from build123d import *

# Parameters (mm, degrees)
SKETCH1_R           = 25
BOSS_EXTRUDE1_DEPTH = 10
SKETCH2_R           = 1.6
CUT_EXTRUDE1_DEPTH  = 37.742346142
SKETCH5_R           = 2.85
CUT_EXTRUDE4_DEPTH  = 3.2
CIRPATTERN1_COUNT   = 4
SKETCH8_R           = 1.6
CUT_EXTRUDE6_DEPTH  = 37.742346142
CUT_EXTRUDE2_DEPTH  = 2.6
CIRPATTERN2_COUNT   = 4
SKETCH4_R           = 7
CUT_EXTRUDE3_DEPTH  = 37.742346142
SKETCH6_R           = 1.6
CUT_EXTRUDE5_DEPTH  = 37.742346142
CIRPATTERN3_COUNT   = 4


with BuildPart() as part:
    # Sketch1 → Boss-Extrude1 (new body)
    with BuildSketch(Plane.XY):
        Circle(SKETCH1_R)
    extrude(amount=BOSS_EXTRUDE1_DEPTH)

    # Sketch2 → Cut-Extrude1 (cut, through all)
    with BuildSketch(Plane.XY.offset(10)):
        with Locations((-8.838834765, 8.838834765)):
            Circle(SKETCH2_R)
    cut_extrude1 = extrude(amount=-CUT_EXTRUDE1_DEPTH, mode=Mode.SUBTRACT)

    # Sketch5 → Cut-Extrude4 (cut)
    with BuildSketch(Plane.XY.offset(10)):
        with Locations((-8.838834765, 8.838834765)):
            Circle(SKETCH5_R)
    cut_extrude4 = extrude(amount=-CUT_EXTRUDE4_DEPTH, mode=Mode.SUBTRACT)

    # CirPattern1: Cut-Extrude1, Cut-Extrude4 ×4 about axis
    cirpattern1_axis = Axis((0, 0, 0), (0, 0, 1))
    add([cut_extrude1.rotate(cirpattern1_axis, i * 360 / CIRPATTERN1_COUNT) for i in range(1, CIRPATTERN1_COUNT)], mode=Mode.SUBTRACT)
    add([cut_extrude4.rotate(cirpattern1_axis, i * 360 / CIRPATTERN1_COUNT) for i in range(1, CIRPATTERN1_COUNT)], mode=Mode.SUBTRACT)

    # Sketch8 → Cut-Extrude6 (cut, through all)
    with BuildSketch(Plane(origin=(0, 0, 0), x_dir=(-1, 0, 0), z_dir=(0, 0, -1))):
        with Locations((0, 14)):
            Circle(SKETCH8_R)
    cut_extrude6 = extrude(amount=-CUT_EXTRUDE6_DEPTH, mode=Mode.SUBTRACT)

    # Sketch3 → Cut-Extrude2 (cut)
    with BuildSketch(Plane.XY):
        Polygon((2.85, 12.354551733), (2.85, 15.645448267), (0, 17.290896534), (-2.85, 15.645448267), (-2.85, 12.354551733), (0, 10.709103466), align=None)
    cut_extrude2 = extrude(amount=CUT_EXTRUDE2_DEPTH, mode=Mode.SUBTRACT)

    # CirPattern2: Cut-Extrude6, Cut-Extrude2 ×4 about axis
    cirpattern2_axis = Axis((0, 0, 0), (0, 0, 1))
    add([cut_extrude6.rotate(cirpattern2_axis, i * 360 / CIRPATTERN2_COUNT) for i in range(1, CIRPATTERN2_COUNT)], mode=Mode.SUBTRACT)
    add([cut_extrude2.rotate(cirpattern2_axis, i * 360 / CIRPATTERN2_COUNT) for i in range(1, CIRPATTERN2_COUNT)], mode=Mode.SUBTRACT)

    # Sketch4 → Cut-Extrude3 (cut, through all)
    with BuildSketch(Plane.XY.offset(10)):
        Circle(SKETCH4_R)
    extrude(amount=-CUT_EXTRUDE3_DEPTH, mode=Mode.SUBTRACT)

    # Sketch6 → Cut-Extrude5 (cut, through all)
    with BuildSketch(Plane(origin=(0, 0, 0), x_dir=(-1, 0, 0), z_dir=(0, 0, -1))):
        with Locations((15.202795796, 15.202795796)):
            Circle(SKETCH6_R)
    cut_extrude5 = extrude(amount=-CUT_EXTRUDE5_DEPTH, mode=Mode.SUBTRACT)

    # CirPattern3: Cut-Extrude5 ×4 about axis
    cirpattern3_axis = Axis((0, 0, 0), (0, 0, 1))
    for i in range(1, CIRPATTERN3_COUNT):
        add(cut_extrude5.rotate(cirpattern3_axis, i * 360 / CIRPATTERN3_COUNT), mode=Mode.SUBTRACT)


solid = part.part
Check sheet for the modelled part. Datum: model origin and axes. Units: mm. A direction names the side the tool comes from. Give positions to 0.01 mm unless a question says otherwise; leave off trailing zeros. Write each loop counter-clockwise with the first axis right and the second up, starting at its lowest first coordinate (ties: lowest second). Pieces come first, ordered by that corner, then holes. Notation, with made-up numbers: (77.25, 54.25) -> (106.25, 54.25) arc R12 cw to (106.25, 75.25) -> close; hole circle Ø1 at (-0.5, 2). An arc over 180 degrees is marked (long way). Use one line per item in the form item = value. Start each with the question number.
1. Access from +Z, -Z, +X, -X, +Y, -Y to the whole of each face (thin tool, end or side, straight path). Record for faces 1 (the cylindrical face through (-16.73, 15.68, 4.93)), 2 (the flat face through (-1, 16, 2.6)).
2. Thickness scan on line 1 along Y through (x, z) = (0, 7.5); line 2 along X through (y, z) = (16.5, 1); line 3 along Y through (x, z) = (16, 1.75). Record the ranges inside material, lowest first. Write a range as from..to.
3. Go/stop test with flat-tipped pins: P1, Ø6, axis at x = 8, z = 3.5, coming from the +Y side; P2, Ø3, axis at x = -13, y = 0.5, coming from the -Z side; P3, Ø3, axis at x = 14, z = 1.5, coming from the +Y side. Record where each tip stops, or that it passes through.
4. Section check C-C (x = 19). Record the cut outline in (y, z), and give its area (3 significant figures).
5. Mould release check, pull along X, two halves, no side actions. Record for faces 3 (the cylindrical face through (23.846, 7.509, 4.93)), 4 (the flat face through (1.44, -11.54, 1.28)): pulls with the +X half, pulls with the -X half, needs draft (parallel to the pull), parting line crosses it, or undercut.
6. Section check B-B (y = 21.5). Record the cut outline in (x, z).
7. Section check A-A (z = 5.75). Count the separate pieces of the cut face and the enclosed holes in it, and give its area (3 significant figures).
Conclusion:
q1.face_1 = +Z, -Z
q1.face_2 = -Z
q2.line_1 = -25..-15.6, -12.4..-7, 7..12.4, 15.6..25
q2.line_2 = -18.78..-16.14, -14.27..-1.37, 1.37..14.27, 16.14..18.78
q2.line_3 = -19.21..-16.59, -13.82..-2.24, 2.24..13.82, 16.59..19.21
q3.P1 = 24.49
q3.P2 = 2.6
q3.P3 = 21.65
q4.outline = (-16.25, 0) -> (16.25, 0) -> (16.25, 10) -> (-16.25, 10) -> close
q4.area = 325 mm²
q5.face_3 = parting line crosses it
q5.face_4 = undercut
q6.outline = (-12.76, 0) -> (12.76, 0) -> (12.76, 10) -> (-12.76, 10) -> close
q7.separate_pieces = 1
q7.enclosed_holes = 13
q7.area = 1,710 mm²
